Build history of the part. All positions in model axes, mm. A direction names the side the tool comes from. Give positions to 0.01 mm unless a question says otherwise; leave off trailing zeros. Order: outer loops, then holes, each group sorted by start corner. A loop starts at its lowest first (then second) coordinate and runs counter-clockwise, first axis right, second up. Notation, with made-up numbers: (57.25, 31.25) - (105.25, 31.25) arc R24 ccw to (105.25, 69.25) - close; hole circle Ø9 at (64, 2). An arc over 180 degrees is marked (long way). One line per item, written item: value.
```python
from build123d import *

# Parameters (mm, degrees)
F2_SIZE2 = 2
F2_SIZE  = 2


with BuildPart() as f1:
    # F0 (on Front) → F1 (revolve)
    with BuildSketch(Plane.XZ):
        Polygon((0, 80), (0, 0), (21, 0), (21, 25), (14, 25), (14, 37), (9, 37), (9, 40), (11, 40), (11, 80), align=None)
    revolve(axis=Axis((0, 0, 40), (0, 0, -1)))

    # F2
    f2_edges = [f1.edges().sort_by_distance(p)[0] for p in [
        (-11, 0, 80),
        (-21, 0, 0),
    ]]
    chamfer(f2_edges, length=F2_SIZE, length2=F2_SIZE2)


solid = f1.part
```
(1) Slice it at C-C, the plane z = 16.5. Give the cut face in (x, y), and give its area (3 significant figures).
Completed:
outline: circle Ø42 at (0, 0)
area: 1,390 mm²
(2) Pin check, flat tips, straight feed: P1, Ø6, axis at y = -10.5, z = 71, coming from the +X side; P2, Ø2, axis at y = -10, z = 9, coming from the -X side; P3, Ø2, axis at x = -15, y = 14, coming from the +Z side. Stop position of each tip, or through.
Completed:
P1: x = 8.05
P2: x = -18.97
P3: z = 25
(3) 3-axis set-ups, long thin cutter, end or side, ignore diameter. For faces 1 (the face through (-2.38, 10.74, 59.27)), 2 (the face through (9, 3, 37)), 3 (the face through (20.03, -6.31, 13.66)): which of +Z, -Z, +X, -X, +Y, -Y reach the whole face in a straight line?
Completed:
face 1: +Z
face 2: none
face 3: +Z, -Z
(4) Drill centre lines: line 1 (Z direction, x = -9, y = 11); line 2 (Y direction, x = 0, z = 38); line 3 (Z direction, x = 8, y = 7.5). Where is each one in solid material? Low to high.
Completed:
line 1: 0 to 25
line 2: -9 to 9
line 3: 0 to 37, 40 to 78.03
(5) Pull direction Z, two halves, no side cores. Call faces 4 (the face through (0, 0, 80)), 5 (the face through (12.932, 5.362, 31.084)), 6 (the face through (-2, 9, 40)): +Z half, -Z half, draft (parallel to the pull), parting line (faces both ways), or undercut.
Completed:
face 4: +Z half
face 5: draft
face 6: undercut
(6) Slice it at D-D, the plane z = 55. Give the cut face in (x, y), and give its area (3 significant figures).
Completed:
outline: circle Ø22 at (0, 0)
area: 380 mm²
(7) Slice it at A-A, the plane y = 0. Give the cut face in (x, z).
Completed:
outline: (-21, 2) - (-19, 0) - (19, 0) - (21, 2) - (21, 25) - (14, 25) - (14, 37) - (9, 37) - (9, 40) - (11, 40) - (11, 78) - (9, 80) - (-9, 80) - (-11, 78) - (-11, 40) - (-9, 40) - (-9, 37) - (-14, 37) - (-14, 25) - (-21, 25) - close
